Geometry: final body of the model. Coordinates: model frame, mm. Coordinates: 2 decimals unless noted, no trailing zeros. Loops run counter-clockwise (first coordinate to the right, second up) from the corner with the lowest first, then second, coordinate; pieces in that order, holes last. Notation, with made-up numbers: (55.25, -15.5) - (85.25, -15.5) arc R32 cw to (85.25, 13.5) - close; hole circle Ø2 at (11.5, -15). An arc over 180 degrees is marked (long way). Return JSON: item names as keys, results as strings.
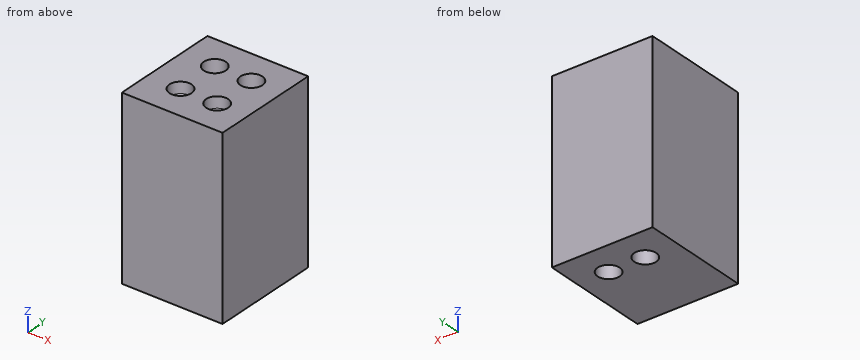
from build123d import *

# Parameters (mm, degrees)
F0_W     = 22.9004416908
F0_H     = 25
F0_R     = 2.5
F1_DEPTH = 40
F2_DEPTH = 40
F3_DEPTH = 5
F4_R     = 2.5


# Not quite as in the source:
# - a feature names something its author has since deleted; it is built from what else it names


with BuildPart() as f1:
    # F0 (on Top) → F1 (new body)
    with BuildSketch(Plane.XY):
        with Locations((-31.441590436, 3.4210662183)):
            Rectangle(F0_W, F0_H)
        with Locations((-35.3918112814, -1.5789337817)):
            Circle(F0_R, mode=Mode.SUBTRACT)
        with Locations((-27.0588112814, -1.5789337817)):
            Circle(F0_R, mode=Mode.SUBTRACT)
        with Locations((-35.3918112814, 8.4210662183)):
            Circle(F0_R, mode=Mode.SUBTRACT)
        with Locations((-27.0588112814, 8.4210662183)):
            Circle(F0_R, mode=Mode.SUBTRACT)
        with Locations((-35.3918112814, 8.4210662183)):
            Circle(F0_R)
        with Locations((-27.0588112814, 8.4210662183)):
            Circle(F0_R)
        with Locations((-27.0588112814, -1.5789337817)):
            Circle(F0_R)
        with Locations((-35.3918112814, -1.5789337817)):
            Circle(F0_R)
    extrude(amount=-F1_DEPTH)

    # F0 (on Top) → F2 (cut)
    with BuildSketch(Plane.XY):
        with Locations((-35.3918112814, 8.4210662183)):
            Circle(F0_R)
        with Locations((-27.0588112814, 8.4210662183)):
            Circle(F0_R)
    extrude(amount=-F2_DEPTH, mode=Mode.SUBTRACT)

    # F0 (on Top) → F3 (cut)
    with BuildSketch(Plane.XY):
        with Locations((-35.3918112814, -1.5789337817)):
            Circle(F0_R)
        with Locations((-27.0588112814, -1.5789337817)):
            Circle(F0_R)
    extrude(amount=-F3_DEPTH, mode=Mode.SUBTRACT)

    # F4
    f4_edges = [f1.edges().sort_by_distance(p)[0] for p in [
        (-37.891811, -1.578934, -5),
        (-29.558811, -1.578934, -5),
    ]]
    fillet(f4_edges, radius=F4_R)


solid = f1.part
Item 1: Section query C-C, the plane y = -2. Return loops of the section in (x, z), and give its area (3 significant figures).
Worked out:
{"outline": "(-42.89, -40) - (-19.99, -40) - (-19.99, 0) - (-24.59, 0) - (-24.59, -2.5) arc R2.46 cw to (-29.52, -2.5) - (-29.52, 0) - (-32.93, 0) - (-32.93, -2.5) arc R2.46 cw to (-37.86, -2.5) - (-37.86, 0) - (-42.89, 0) - close", "area": "872 mm^2"}
Item 2: First-contact query: pin 1 Ø4.5 at (x, y) = (-35.39, -1.58) entering from +Z; pin 2 Ø3 at (x, y) = (-27.06, 8.42) entering from -Z. Flat tips, straight axial feed; report the tip coordinate or a pass-through.
Worked out:
{"pin 1": "z = -3.59", "pin 2": "through"}
Item 3: Section query A-A, the plane y = 7. Return loops of the section in (x, z).
Worked out:
{"outline": "(-42.89, -40) - (-37.45, -40) - (-37.45, 0) - (-42.89, 0) - close; (-33.33, -40) - (-29.12, -40) - (-29.12, 0) - (-33.33, 0) - close; (-25, -40) - (-19.99, -40) - (-19.99, 0) - (-25, 0) - close"}
Item 4: Section query B-B, the plane z = -18. Return loops of the section in (x, y).
Worked out:
{"outline": "(-42.89, -9.08) - (-19.99, -9.08) - (-19.99, 15.92) - (-42.89, 15.92) - close; hole circle Ø5 at (-35.39, 8.42); hole circle Ø5 at (-27.06, 8.42)"}
Item 5: Ray query, probe 1 along X at (y, z) = (8.5, -17.5); probe 2 along X at (y, z) = (7.5, -11.5); probe 3 along Z at (x, y) = (-25.75, -1.75). Return the intervals inside material, ascending. Write a range as from..to.
Worked out:
{"probe 1": "-42.89..-37.89, -32.89..-29.56, -24.56..-19.99", "probe 2": "-42.89..-37.72, -33.07..-29.38, -24.73..-19.99", "probe 3": "-40..-4.62"}
